Verification items for this drawing (mm, ordinates from the low corner). A direction names the side the tool comes from. Round coordinates to 2 decimals unless told otherwise and drop trailing zeros. Loops run counter-clockwise (first coordinate to the right, second up) from the corner with the lowest first, then second, coordinate; pieces in that order, holes last. Notation, with made-up numbers: (14.25, 62) -> (42.25, 62) arc R22 ccw to (42.25, 90) -> close; hole circle Ø6 at (69.25, 89). An arc over 180 degrees is marked (long way). Use a Markdown table: item, result. Add a question column.
Q1. Set-up check for the marked faces 4, 5 and 6: record each of +Z, -Z, +X, -X, +Y, -Y from which the full face is reachable in a straight line by a thin tool's end or side.
Q2. Gauge pin test, flat ends, axial feed: P1, Ø1, axis at x = 58, y = 2.5, coming from the -Z side; P2, Ø3.5, axis at x = 98.68, z = 62.77, coming from the -Y side; P3, Ø1.5, axis at x = 61.5, z = 56.5, coming from the +Y side; P4, Ø20.5, axis at x = 62, z = 11.5, coming from the +Y side. Record the tip position at first contact, or that the pin passes through.
Q3. Sectioned sample at B-B, the plane z = 57.5. Enter the section's corners in (x, y).
Q4. Release check for a two-part mould opening along Z. For the marked faces 1, 2 and 3 record: released by +Z, released by -Z, zero draft, split by the parting line, or undercut.
Q5. Sectioned sample at D-D, the plane z = 22. Enter the section's corners in (x, y).
Q6. Material ranges on L1, parallel to X at y = 4.25, z = 35; L2, parallel to Y at x = 58, z = 15; L3, parallel to Y at x = 19, z = 51, recorded low to high.
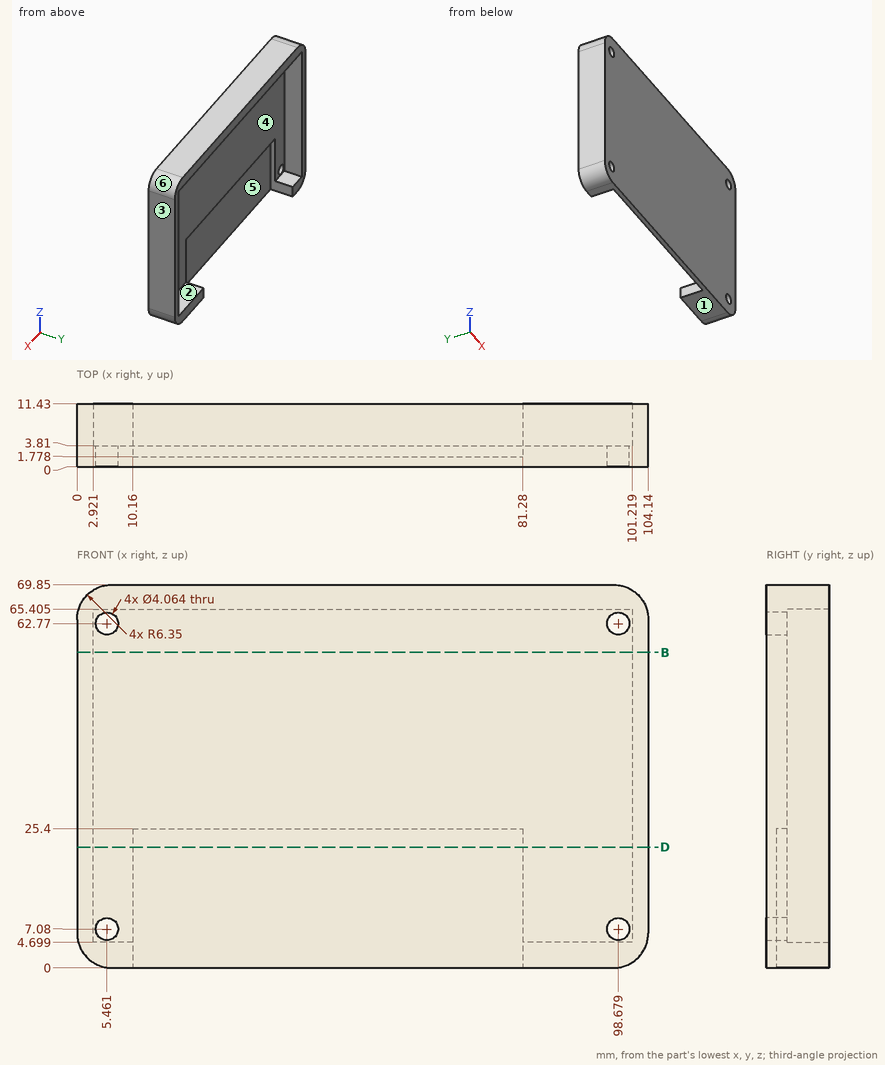
Values:
| question | item | result |
|---|---|---|
| 1 | face 4 | +Y |
| 1 | face 5 | -Z, +Y |
| 1 | face 6 | +Z, +X, +Y, -Y |
| 2 | P1 | z = 25.4 |
| 2 | P2 | through |
| 2 | P3 | y = 3.81 |
| 2 | P4 | y = 1.78 |
| 3 | outline | (0, 0) -> (104.14, 0) -> (104.14, 11.43) -> (101.22, 11.43) -> (101.22, 3.81) -> (2.92, 3.81) -> (2.92, 11.43) -> (0, 11.43) -> close |
| 4 | face 1 | released by -Z |
| 4 | face 2 | undercut |
| 4 | face 3 | zero draft |
| 5 | outline | (0, 0) -> (104.14, 0) -> (104.14, 11.43) -> (101.22, 11.43) -> (101.22, 3.81) -> (81.28, 3.81) -> (81.28, 1.78) -> (10.16, 1.78) -> (10.16, 3.81) -> (2.92, 3.81) -> (2.92, 11.43) -> (0, 11.43) -> close |
| 6 | L1 | 0 to 2.92, 101.22 to 104.14 |
| 6 | L2 | 0 to 1.78 |
| 6 | L3 | 0 to 3.81 |
